The drawing under review shows one solid part. Ordinate dimensions are in mm from its lowest x, y, z. A direction names the side the tool comes from. Coordinates: 2 decimals unless noted, no trailing zeros. Write each loop counter-clockwise with the first axis right and the second up, starting at its lowest first coordinate (ties: lowest second). Pieces come first, ordered by that corner, then holes.
1) We need section A-A on z = 25. Write out the cut boundary in (x, y), then the cut area to 3 significant figures.
2) For the marked faces 4 and 5, list the 3-axis set-ups (+Z, -Z, +X, -X, +Y, -Y) from which the entire face can be reached by the end or side of a thin tool; tool diameter is ignored.
3) Insertion check: P1, Ø10, axis at y = 4, z = 29, coming from the +X side; P2, Ø5, axis at y = 2.5, z = 33.5, coming from the +X side; P3, Ø4, axis at y = 21.5, z = 19.5, coming from the +X side. Each pin has a flat end and moves straight along its axis. Give the tip position at first contact, or say it passes through.
4) We need section C-C on y = 21.25. Write out the cut boundary in (x, z), then the cut area to 3 significant figures.
5) To check wall thickness, follow line 1 along X through (y, z) = (7.75, 25); line 2 along X through (y, z) = (18, 25); line 3 along Z through (x, y) = (5, 23). State the ranges of each line that lie inside material, in increasing order.
6) Mouldability with a two-part tool opening along X and no side actions: class the marked faces 1, 2 and 3 as pulls with the +X half, pulls with the -X half, needs draft (parallel to the pull), parting line crosses it, or undercut.
7) We need section B-B on y = 10.75. Write out the cut boundary in (x, z), then the cut area to 3 significant figures.
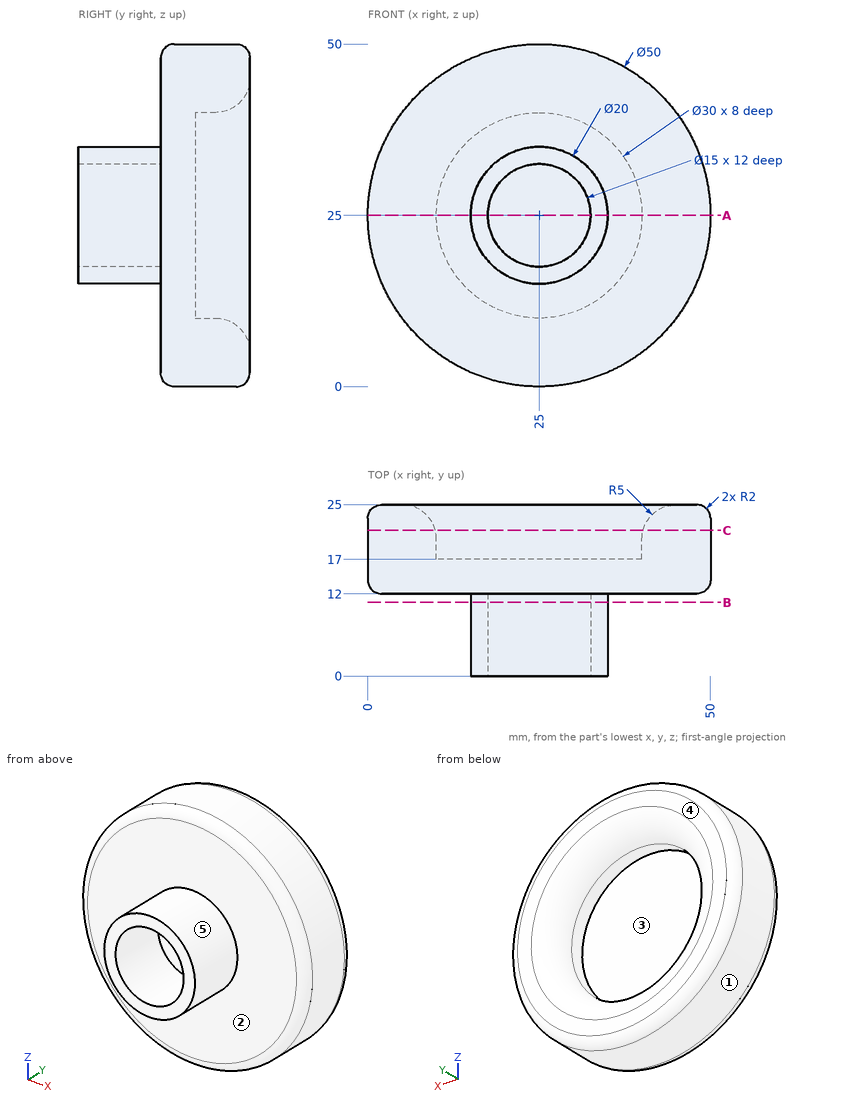
Result:
1. outline: (0, 14) arc R2 ccw to (2, 12) - (15, 12) - (15, 0) - (17.5, 0) - (17.5, 12) - (32.5, 12) - (32.5, 0) - (35, 0) - (35, 12) - (48, 12) arc R2 ccw to (50, 14) - (50, 23) arc R2 ccw to (48, 25) - (45, 25) arc R5 ccw to (40, 20) - (40, 17) - (10, 17) - (10, 20) arc R5 ccw to (5, 25) - (2, 25) arc R2 ccw to (0, 23) - close
1. area: 456 mm2
2. face 4: +Z, -Z, +X, -X, +Y
2. face 5: -Y
3. P1: stops at x = 35
3. P2: stops at x = 33
3. P3: stops at x = 49.75
4. outline: circle Ø50 at (25, 25); hole circle Ø30.32 at (25, 25)
4. area: 1,240 mm2
5. line 1: x = 15 to 17.5, 32.5 to 35
5. line 2: x = 0 to 10, 40 to 50
5. line 3: z = 10 to 40
6. face 1: parting line crosses it
6. face 2: needs draft
6. face 3: undercut
7. outline: circle Ø20 at (25, 25); hole circle Ø15 at (25, 25)
7. area: 137 mm2
